Autodesk Inventor part; units mm, degrees
ref_plane "YZ Plane" through (0, 0, 0) normal (1, 0, 0) x (0, 1, 0)
ref_plane "XZ Plane" through (0, 0, 0) normal (0, 1, 0) x (-1, 0, 0)
ref_plane "XY Plane" through (0, 0, 0) normal (0, 0, 1) x (1, 0, 0)
sketch "Sketch1" plane through (0, 0, 0) normal (0, 1, 0) x (-1, 0, 0)
  line L0 (232.1908, -176.5808) -> (232.1908, -3.7592)
  arc A0 (232.1908, -3.7592) -> (227.4316, 1) centre (227.4316, -3.7592) ccw
  line L1 (227.4316, 1) -> (0, 1)
  arc A1 (0, 1) -> (-4.7592, -3.7592) centre (0, -3.7592) ccw
  arc A2 (-4.7592, -176.5808) -> (0, -181.34) centre (0, -176.5808) ccw
  arc A3 (227.4316, -181.34) -> (232.1908, -176.5808) centre (227.4316, -176.5808) ccw
  circle A4 centre (130, -129.34) radius 2.25
  circle A5 centre (129.9861, -89.34) radius 2.25
  circle A6 centre (90, -129.34) radius 2.25
  circle A7 centre (89.9861, -89.34) radius 2.25
  circle A8 centre (180, -110) radius 2.75
  circle A9 centre (55, -110) radius 2.75
  circle A10 centre (90, -45) radius 3
  circle A11 centre (190, -45) radius 3
  circle A12 centre (190, -65) radius 3
  circle A13 centre (90, -65) radius 3
  circle A14 centre (140, -45) radius 3
  circle A15 centre (40, -45) radius 3
  circle A16 centre (140, -65) radius 3
  circle A17 centre (40, -65) radius 3
  line L2 (230.1908, -176.5808) -> (230.1908, -3.7592)
  arc A18 (230.1908, -3.7592) -> (227.4316, -1) centre (227.4316, -3.7592) ccw
  line L3 (227.4316, -1) -> (0, -1)
  arc A19 (0, -1) -> (-2.7592, -3.7592) centre (0, -3.7592) ccw
  arc A20 (-2.7592, -176.5808) -> (0, -179.34) centre (0, -176.5808) ccw
  arc A21 (227.4316, -179.34) -> (230.1908, -176.5808) centre (227.4316, -176.5808) ccw
  line L4 (-4.7592, -3.7592) -> (-4.7592, -176.5808)
  line L5 (-2.7592, -3.7592) -> (-2.7592, -176.5808)
  line L6 (0, -179.34) -> (227.4316, -179.34)
  line L7 (227.4316, -181.34) -> (0, -181.34)
  line L8 (0, 0) -> (0, -15)
  line L9 (0, 0) -> (15, 0) construction
  line L10 (0, 0) -> (15, 0)
  line L11 (0, 0) -> (15, 0) construction
  circle A22 centre (15, -135) radius 2.25
  circle A23 centre (73, -135) radius 2.25
  circle A24 centre (15, -77) radius 2.25
  point P0 (230.1908, -3.7592)
  point P1 (0, -1)
  dimension "d0" = 2
  dimension "d1" = 2
  dimension "d2" = 2
  dimension "d3" = 2
  dimension "d5" = 2
  dimension "d7" = 2
  dimension "d8" = 227.4316
  dimension "d9" = 172.8216
  dimension "d10" = 4.7592
  dimension "d45" = 15
  dimension "d46" = 90
  dimension "d47" = 15
  dimension "d48" = 0
  dimension "d49" = 110
  dimension "d50" = 55
  dimension "d51" = 125
  dimension "d52" = 110
  dimension "d54" = 40
  dimension "d55" = 40
  dimension "d56" = 40
  dimension "d57" = 40
  dimension "d58" = 50
  dimension "d59" = 100.1908
  dimension "d60" = 2.7592
  dimension "d61" = 1
  dimension "d62" = 4.7592
  dimension "d63" = 178.34
  dimension "d64" = 180.34
  dimension "d65" = 172.8216
  dimension "d66" = 230.1908
  dimension "d67" = 4.5
  dimension "d68" = 5.5
  dimension "d69" = 6
  dimension "d70" = 40.1908
  dimension "d71" = 64
  dimension "d72" = 20
  dimension "d73" = 50
  dimension "d74" = 50
  dimension "d75" = 50
  dimension "d76" = 20
  dimension "d77" = 20
  dimension "d78" = 20
  dimension "d79" = 50
  dimension "d87" = 4.5
  dimension "d89" = 25
  dimension "d90" = 40
  dimension "d91" = 4.5
  dimension "d92" = 58
  dimension "d93" = 4.5
  dimension "d94" = 58
extrude "Extrusion1" add sketch "Sketch1" along normal blind 6 contours A21 L6 A20 L5 A19 L3 A18 L2
sketch "Sketch2" plane through (0, 6, 0) normal (0, 1, 0) x (1, 0, 0)
  line L0 (-232.1908, 176.5808) -> (-232.1908, 3.7592)
  arc A0 (-232.1908, 3.7592) -> (-227.4316, -1) centre (-227.4316, 3.7592) ccw
  line L1 (-227.4316, -1) -> (0, -1)
  arc A1 (0, -1) -> (4.7592, 3.7592) centre (0, 3.7592) ccw
  arc A2 (4.7592, 176.5808) -> (0, 181.34) centre (0, 176.5808) ccw
  arc A3 (-227.4316, 181.34) -> (-232.1908, 176.5808) centre (-227.4316, 176.5808) ccw
  circle A4 centre (-130, 135) radius 2
  circle A5 centre (-130, 95) radius 2
  circle A6 centre (-90, 135) radius 2
  circle A7 centre (-90, 95) radius 2
  circle A8 centre (-160.0797, 100) radius 2.75
  circle A9 centre (-60.0797, 100) radius 2.75
  circle A10 centre (-90, 45) radius 2.5
  circle A11 centre (-190, 45) radius 2.5
  circle A12 centre (-190, 65) radius 2.5
  circle A13 centre (-90, 65) radius 2.5
  circle A14 centre (-140, 45) radius 2.5
  circle A15 centre (-40, 45) radius 2.5
  circle A16 centre (-140, 65) radius 2.5
  circle A17 centre (-40, 65) radius 2.5
  line L2 (-230.1908, 176.5808) -> (-230.1908, 3.7592)
  arc A18 (-230.1908, 3.7592) -> (-227.4316, 1) centre (-227.4316, 3.7592) ccw
  line L3 (-227.4316, 1) -> (0, 1)
  arc A19 (0, 1) -> (2.7592, 3.7592) centre (0, 3.7592) ccw
  arc A20 (2.7592, 176.5808) -> (0, 179.34) centre (0, 176.5808) ccw
  arc A21 (-227.4316, 179.34) -> (-230.1908, 176.5808) centre (-227.4316, 176.5808) ccw
  line L4 (4.7592, 3.7592) -> (4.7592, 176.5808)
  line L5 (2.7592, 3.7592) -> (2.7592, 176.5808)
  line L6 (0, 179.34) -> (-227.4316, 179.34)
  line L7 (-227.4316, 181.34) -> (0, 181.34)
  line L8 (0, 179.34) -> (-227.4316, 179.34)
  line L9 (-113.7158, 179.34) -> (-113.7158, 1)
  line L10 (-227.4316, 1) -> (0, 1)
  line L11 (-118.7158, 120.17) -> (-108.7158, 120.17)
  line L12 (-108.7158, 120.17) -> (-108.7158, 60.17)
  line L13 (-108.7158, 60.17) -> (-118.7158, 60.17)
  line L14 (-118.7158, 60.17) -> (-118.7158, 120.17)
  line L15 (-118.7158, 120.17) -> (-108.7158, 60.17) construction
  line L16 (-108.7158, 120.17) -> (-118.7158, 60.17) construction
  line L17 (-113.7158, 179.34) -> (-113.7158, 159.34)
  line L18 (2.7592, 139.34) -> (-230.1908, 139.34)
  line L19 (-230.1908, 139.34) -> (-230.1908, 179.34)
  line L20 (-230.1908, 179.34) -> (2.7592, 179.34)
  line L21 (2.7592, 179.34) -> (2.7592, 139.34)
  line L22 (2.7592, 139.34) -> (-230.1908, 179.34) construction
  line L23 (-230.1908, 139.34) -> (2.7592, 179.34) construction
  line L24 (-113.7158, 1) -> (-113.7158, 16)
  line L25 (-230.1908, 31) -> (2.7592, 31)
  line L26 (2.7592, 31) -> (2.7592, 1)
  line L27 (2.7592, 1) -> (-230.1908, 1)
  line L28 (-230.1908, 1) -> (-230.1908, 31)
  line L29 (-230.1908, 31) -> (2.7592, 1) construction
  line L30 (2.7592, 31) -> (-230.1908, 1) construction
  line L31 (-227.4316, 1) -> (0, 1)
  line L32 (-230.1908, 179.34) -> (-200.1908, 179.34)
  line L33 (-200.1908, 179.34) -> (-200.1908, 1)
  line L34 (-200.1908, 1) -> (-230.1908, 1)
  line L35 (-230.1908, 1) -> (-230.1908, 179.34)
  line L36 (2.7592, 1) -> (-7.2408, 1)
  line L37 (-7.2408, 1) -> (-7.2408, 179.34)
  line L38 (-7.2408, 179.34) -> (2.7592, 179.34)
  line L39 (2.7592, 179.34) -> (2.7592, 1)
  point P0 (230.1908, -176.5808)
  point P1 (230.1908, -3.7592)
  point P2 (227.4316, -1)
  point P3 (0, -1)
  point P4 (0, 0)
  point P5 (230.1908, -176.5808)
  point P6 (230.1908, -3.7592)
  point P7 (227.4316, -1)
  point P8 (0, -1)
  point P9 (-113.7158, 90.17)
  point P10 (-113.7158, 120.17)
  point P11 (-113.7158, 60.17)
  point P12 (-113.7158, 1)
  point P13 (0, 1)
  point P14 (-230.1908, 3.7592)
  point P15 (-227.4316, 1)
  point P16 (-113.7158, 139.34)
  point P17 (-7.2408, 139.34)
  point P18 (-7.2408, 31)
  point P19 (-113.7158, 31)
  dimension "d22" = 2
  dimension "d23" = 2
  dimension "d24" = 2
  dimension "d25" = 2
  dimension "d26" = 2
  dimension "d27" = 2
  dimension "d28" = 227.4316
  dimension "d29" = 172.8216
  dimension "d30" = 4.7592
  dimension "d31" = 10
  dimension "d32" = 60
  dimension "d37" = 20
  dimension "d38" = 40
  dimension "d39" = 15
  dimension "d40" = 30
  dimension "d41" = 30
  dimension "d42" = 10
extrude "Extrusion3" cut sketch "Sketch2" against normal through all contours A4 | A5 | A8 | A11 | A12 | A14 | A16 | A21 L6 L33 L18 L2 | L18 L33 L25 L2 | L25 L33 L3 A18 L2 | L33 L6 L9 L18 | L18 L9 L11 L14 L13 L25 L33 | L25 L9 L3 L33 | L9 L6 L37 L18 | L25 L37 L3 L9 | L37 L6 A20 L5 L18 | L18 L5 L25 L37 | L25 L5 A19 L3 L37
fillet "Fillet3" radius 2 6 edges at (-113.7158, 3, -31) (-118.7158, 3, -60.17) (-118.7158, 3, -120.17) (-7.2408, 3, -31) (-7.2408, 3, -139.34) (-113.7158, 3, -139.34)
equation "\"d1\" = d0"
equation "\"d2\" = d0"
equation "\"d3\" = d0"
equation "\"d5\" = d0"
equation "\"d7\" = d0"
equation "\"d23\" = d22"
equation "\"d24\" = d22"
equation "\"d25\" = d22"
equation "\"d26\" = d22"
equation "\"d27\" = d22"
properties part number "EboxBottom_2"
Read the model definition and answer for the solid it produces. Units are mm, in the model's axes. A direction names the side the tool comes from. Coordinates: 2 decimals unless noted, no trailing zeros. Loops run counter-clockwise (first coordinate to the right, second up) from the corner with the lowest first, then second, coordinate; pieces in that order, holes last. Notation, with made-up numbers: (-11, 53.25) -> (-5, 53.25) arc R15 ccw to (-5, 69.25) -> close; hole circle Ø1 at (21.25, 80). An arc over 180 degrees is marked (long way). Answer in a Markdown table with one row per item.
Item 1: A cutting plane is placed at A-A on x = -15. Determine the outline of the cut face in (y, z).
Returned:
| item | result |
|---|---|
| outline | (0, -139.34) -> (6, -139.34) -> (6, -137.25) -> (0, -137.25) -> close; (0, -132.75) -> (6, -132.75) -> (6, -79.25) -> (0, -79.25) -> close; (0, -74.75) -> (6, -74.75) -> (6, -31) -> (0, -31) -> close |
Item 2: A cutting plane is placed at B-B on z = -65. Determine the outline of the cut face in (x, y).
Returned:
| item | result |
|---|---|
| outline | (-118.72, 0) -> (-93, 0) -> (-93, 6) -> (-118.72, 6) -> close; (-87, 0) -> (-43, 0) -> (-43, 6) -> (-87, 6) -> close; (-37, 0) -> (-7.24, 0) -> (-7.24, 6) -> (-37, 6) -> close |
Item 3: A cutting plane is placed at D-D on z = -77. Determine the outline of the cut face in (x, y), plus the area to 3 significant figures.
Returned:
| item | result |
|---|---|
| outline | (-118.72, 0) -> (-17.25, 0) -> (-17.25, 6) -> (-118.72, 6) -> close; (-12.75, 0) -> (-7.24, 0) -> (-7.24, 6) -> (-12.75, 6) -> close |
| area | 642 mm^2 |
Item 4: For faces 1 (the flat face through (-115, 3, -60.17)), 2 (the flat face through (-62, 0, -84)), 3 (the flat face through (-115, 3, -120.17)), determine the directions among +Z, -Z, +X, -X, +Y, -Y from which every point of the face is accessible in a straight line to the end or side of a thin tool.
Returned:
| item | result |
|---|---|
| face 1 | +Z, -X, +Y, -Y |
| face 2 | +Z, -Z, +X, -X, -Y |
| face 3 | -Z, -X, +Y, -Y |
Item 5: Each of these flat-tipped pins is pushed along its axis until it touches: P1, Ø2.5, axis at x = -115.5, y = 2, coming from the -Z side; P2, Ø2.5, axis at x = -114.5, y = 3, coming from the +Z side; P3, Ø3, axis at y = 2.5, z = -130.5, coming from the -X side. Where does it stop, or does it pass through?
Returned:
| item | result |
|---|---|
| P1 | stops at z = -120.17 |
| P2 | stops at z = -31.72 |
| P3 | stops at x = -113.72 |
Item 6: A cutting plane is placed at C-C on y = 2.05. Give the number of separate pieces and of enclosed holes in the cut face, plus the area to 3 significant figures.
Returned:
| item | result |
|---|---|
| separate pieces | 1 |
| enclosed holes | 10 |
| area | 11,600 mm^2 |
Item 7: Straight lines are drawn through the part: line 1 along Z through (x, y) = (-15, 2.55); line 2 along Z through (x, y) = (-90, 1.6); line 3 along Z through (x, y) = (-42.5, 3.95). For each, find the intervals that lie inside material, in ascending order. Write a range as [from, to].
Returned:
| item | result |
|---|---|
| line 1 | z = [-139.34, -137.25], [-132.75, -79.25], [-74.75, -31] |
| line 2 | z = [-139.34, -131.59], [-127.09, -91.59], [-87.09, -68], [-62, -48], [-42, -31] |
| line 3 | z = [-139.34, -66.66], [-63.34, -46.66], [-43.34, -31] |
Item 8: For a pull along Z with two mould halves and no side action, classify faces 4 (the flat face through (-62, 6, -84)), 5 (the cylindrical face through (-14.512, 2.958, -74.804)), 6 (the flat face through (-61, 3, -31)) as released by +Z, released by -Z, zero draft, split by the parting line, or undercut.
Returned:
| item | result |
|---|---|
| face 4 | zero draft |
| face 5 | undercut |
| face 6 | released by +Z |
